The model under review builds one solid part; all positions refer to its coordinate system, in mm. Face numbers are marked on the shaded views. A direction names the side the tool comes from. Coordinates: 2 decimals unless noted, no trailing zeros. Loops run counter-clockwise (first coordinate to the right, second up) from the corner with the lowest first, then second, coordinate; pieces in that order, holes last. Notation, with made-up numbers: M -8,1 L 43,1 A15 ccw 43,8 Z; hole C 57.25,49 d3. An arc over 180 degrees is marked long. Return JSON: item names as keys, results as strings.
```python
from build123d import *

# Parameters (mm, degrees)
BOSS_EXTRUDE1_DEPTH = 701
SKETCH3_R           = 7
CUT_EXTRUDE1_DEPTH  = 14
SKETCH4_R           = 7
CUT_EXTRUDE2_DEPTH  = 14
SKETCH5_R           = 7
CUT_EXTRUDE3_DEPTH  = 14
SKETCH6_R           = 7
BOSS_EXTRUDE2_DEPTH = 10
SKETCH7_R           = 7
CUT_EXTRUDE4_DEPTH  = 14
SKETCH8_R           = 7
CUT_EXTRUDE5_DEPTH  = 14
SKETCH9_R           = 7
CUT_EXTRUDE6_DEPTH  = 14
SKETCH10_R          = 7
CUT_EXTRUDE7_DEPTH  = 10
SKETCH11_W          = 111.127913471
SKETCH11_H          = 701
BOSS_EXTRUDE3_DEPTH = 50


with BuildPart() as part:
    # Sketch2 → Boss-Extrude1 (new body)
    with BuildSketch(Plane.XY):
        with BuildLine():
            Line((-838, 0), (838, 0))
            ThreePointArc((838, 0), (827.375455805, 31.557279357), (799.290407516, 49.4450652))
            Line((799.290407516, 49.4450652), (-811.709592484, 49.4450652))
            Line((-811.709592484, 49.4450652), (-838, 0))
        make_face()
    extrude(amount=BOSS_EXTRUDE1_DEPTH)

    # Sketch3 → Cut-Extrude1 (cut)
    with BuildSketch(Plane.XY.offset(701)):
        with Locations((753, 11.005388452)):
            Circle(SKETCH3_R)
        with Locations((753, 29.441497119)):
            Circle(SKETCH3_R)
        with Locations((-15, 29.441497119)):
            Circle(SKETCH3_R)
        with Locations((-15, 11.005388452)):
            Circle(SKETCH3_R)
    extrude(amount=-CUT_EXTRUDE1_DEPTH, mode=Mode.SUBTRACT)

    # Sketch4 → Cut-Extrude2 (cut)
    with BuildSketch(Plane(origin=(0, 0, 0), x_dir=(-1, 0, 0), z_dir=(0, 0, -1))):
        with Locations((-753, 11)):
            Circle(SKETCH4_R)
        with Locations((-753, 29.4)):
            Circle(SKETCH4_R)
        with Locations((15, 11)):
            Circle(SKETCH4_R)
        with Locations((15, 29.4)):
            Circle(SKETCH4_R)
    extrude(amount=-CUT_EXTRUDE2_DEPTH, mode=Mode.SUBTRACT)

    # Sketch5 → Cut-Extrude3 (cut)
    with BuildSketch(Plane(origin=(0, 0, 0), x_dir=(-1, 0, 0), z_dir=(0, 0, -1))):
        with Locations((-320.866149007, 24.947412588)):
            Circle(SKETCH5_R)
        with Locations((-278.502426445, 24.947412588)):
            Circle(SKETCH5_R)
    extrude(amount=-CUT_EXTRUDE3_DEPTH, mode=Mode.SUBTRACT)

    # Sketch6 → Boss-Extrude2 (add)
    with BuildSketch(Plane(origin=(0, 0, 0), x_dir=(-1, 0, 0), z_dir=(0, 0, -1))):
        with Locations(Location((804.854796242, 24.362661379, 0), (0, 0, 180))):
            Circle(SKETCH6_R)
    extrude(amount=BOSS_EXTRUDE2_DEPTH)

    # Sketch7 → Cut-Extrude4 (cut)
    with BuildSketch(Plane(origin=(0, 0, 0), x_dir=(-1, 0, 0), z_dir=(0, 0, -1))):
        with Locations((-365.57912829, 24.947412588)):
            Circle(SKETCH7_R)
        with Locations((-405.274636015, 24.947412588)):
            Circle(SKETCH7_R)
        with Locations((-458.742054583, 24.947412588)):
            Circle(SKETCH7_R)
        with Locations((-433.628570104, 24.947412588)):
            Circle(SKETCH7_R)
    extrude(amount=-CUT_EXTRUDE4_DEPTH, mode=Mode.SUBTRACT)

    # Sketch8 → Cut-Extrude5 (cut)
    with BuildSketch(Plane.XY.offset(701)):
        with Locations((226.886142598, 21.805746879)):
            Circle(SKETCH8_R)
        with Locations((268.91811361, 21.805746879)):
            Circle(SKETCH8_R)
        with Locations((305.755121912, 21.805746879)):
            Circle(SKETCH8_R)
        with Locations((342.119860878, 21.805746879)):
            Circle(SKETCH8_R)
        with Locations((407.293029413, 21.805746879)):
            Circle(SKETCH8_R)
        with Locations((439.819163205, 21.805746879)):
            Circle(SKETCH8_R)
        with Locations((478.174989696, 21.805746879)):
            Circle(SKETCH8_R)
    extrude(amount=-CUT_EXTRUDE5_DEPTH, mode=Mode.SUBTRACT)

    # Sketch9 → Cut-Extrude6 (cut)
    with BuildSketch(Plane.XY.offset(701)):
        with Locations((-804.854796242, 22.721056166)):
            Circle(SKETCH9_R)
    extrude(amount=-CUT_EXTRUDE6_DEPTH, mode=Mode.SUBTRACT)

    # Sketch10 → Cut-Extrude7 (cut)
    with BuildSketch(Plane.XY.offset(701)):
        with Locations((342.119860878, 21.805746879)):
            Circle(SKETCH10_R)
        with Locations((359.619860878, 21.805746879)):
            Circle(SKETCH10_R)
    extrude(amount=-CUT_EXTRUDE7_DEPTH, mode=Mode.SUBTRACT)

    # Sketch11 → Boss-Extrude3 (add)
    with BuildSketch(Plane(origin=(0, 49.4450652, 0), x_dir=(1, 0, 0), z_dir=(0, 1, 0))):
        with Locations((-756.145635749, -350.5)):
            Rectangle(SKETCH11_W, SKETCH11_H)
    extrude(amount=BOSS_EXTRUDE3_DEPTH)


solid = part.part
```
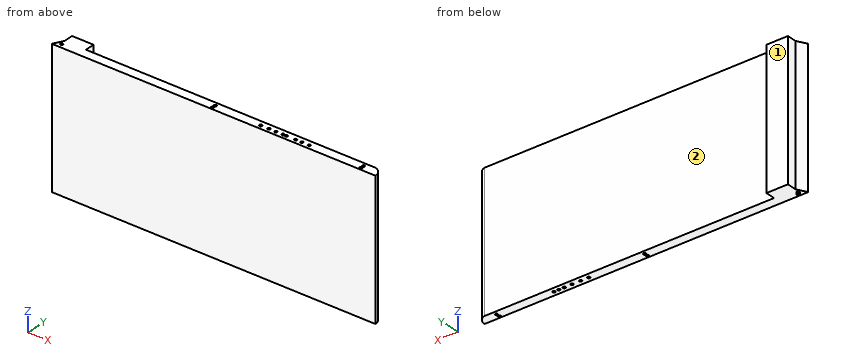
1. Add section B-B on x = 611.5. Give the boundary of the cut face in (y, z).
Check values:
{"outline": "M 0,0 L 49.45,0 L 49.45,701 L 0,701 Z"}
2. Machinability: for the marked faces 1 and 2, which of the approach directions +Z, -Z, +X, -X, +Y, -Y give a long, thin tool a straight path to every point of the face, cutting with its end or side? Answer none if there is none.
Check values:
{"face 1": "+Z, -Z, +X, -X, +Y", "face 2": "+Z, -Z, +X, +Y"}
3. To check wall thickness, follow line 1 (Y direction, x = 753, z = 6); line 2 (Y direction, x = -71, z = 28); line 3 (X direction, y = 68.5, z = 603). State the ranges of each line that lie inside material, in increasing order.
Check values:
{"line 1": "0 to 4, 18 to 22.4, 36.4 to 49.45", "line 2": "0 to 49.45", "line 3": "-811.71 to -700.58"}
4. Insertion check: pin 1 Ø6 at (y, z) = (63.5, 422.5) entering from +X; pin 2 Ø2 at (x, y) = (495.5, 39.5) entering from -Z; pin 3 Ø8 at (x, z) = (-15, 330) entering from +Y; pin 4 Ø1 at (x, z) = (-171, 208.5) entering from -Y. Each pin has a flat end and moves straight along its axis. Give the tip position at first contact, or say it passes through.
Check values:
{"pin 1": "x = -700.58", "pin 2": "z = 0", "pin 3": "y = 49.45", "pin 4": "y = 0"}
5. Add section A-A on z = 414.5. Give the boundary of the cut face in (x, y), plus the area to 3 significant figures.
Check values:
{"outline": "M -838,0 L 838,0 A50 ccw 799.29,49.45 L -700.58,49.45 L -700.58,99.45 L -811.71,99.45 L -811.71,49.45 Z", "area": "87,300 mm²"}
